Build history of the part. All positions in model axes, mm. Round coordinates to 2 decimals unless told otherwise and drop trailing zeros. Write each loop counter-clockwise with the first axis right and the second up, starting at its lowest first coordinate (ties: lowest second). Pieces come first, ordered by that corner, then holes. Notation, with made-up numbers: M -2,33 L 25,33 A22 ccw 25,72 Z; hole C -32,-23.75 d2. An arc over 180 degrees is marked long. Write item = value, one per line.
from build123d import *

# Parameters (mm, degrees)
BOSS_EXTRUDE1_DEPTH = 3
SKETCH2_R           = 1.5
SKETCH2_W           = 6
SKETCH2_H           = 4
CUT_EXTRUDE1_DEPTH  = 3


with BuildPart() as part:
    # Sketch1 → Boss-Extrude1 (new body)
    with BuildSketch(Plane(origin=(0, 0, 0), x_dir=(1, 0, 0), z_dir=(0, 1, 0))):
        Polygon((-41, -41), (-17.5, -41), (-17.5, -38), (17.5, -38), (17.5, -41), (41, -41), (41, -17.5), (38, -17.5), (38, 17.5), (41, 17.5), (41, 41), (17.5, 41), (17.5, 38), (-17.5, 38), (-17.5, 41), (-41, 41), (-41, 17.5), (-38, 17.5), (-38, -17.5), (-41, -17.5), align=None)
    extrude(amount=BOSS_EXTRUDE1_DEPTH)

    # Sketch2 → Cut-Extrude1 (cut)
    with BuildSketch(Plane(origin=(0, 3, 0), x_dir=(1, 0, 0), z_dir=(0, 1, 0))):
        with Locations((0, -5.5)):
            Circle(SKETCH2_R)
        with Locations((0, 12)):
            Rectangle(SKETCH2_W, SKETCH2_H)
    extrude(amount=-CUT_EXTRUDE1_DEPTH, mode=Mode.SUBTRACT)


solid = part.part
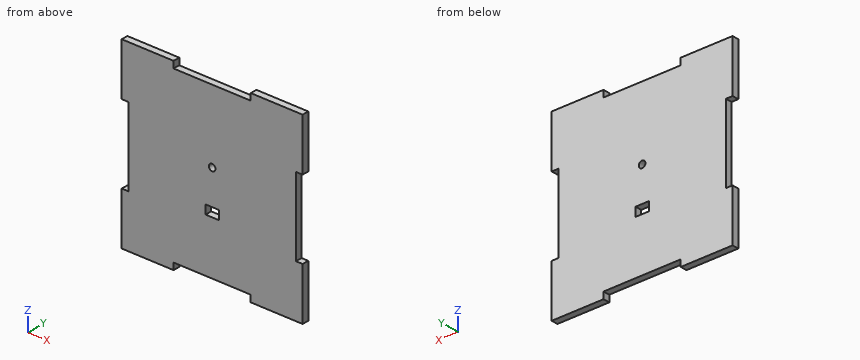
1. Band-saw the part on B-B (x = 0). List the corners of the cut face in (y, z).
Responses:
outline = M 0,-38 L 3,-38 L 3,-14 L 0,-14 Z; M 0,-10 L 3,-10 L 3,4 L 0,4 Z; M 0,7 L 3,7 L 3,38 L 0,38 Z
2. Probe probe 1 along Z at (x, y) = (0, 1.6); probe 2 along X at (y, z) = (2.3, 5.5); probe 3 along Z at (x, y) = (-2.5, 1). List the from-to ranges inside material, lowest first.
Responses:
probe_1 = -38 to -14, -10 to 4, 7 to 38
probe_2 = -38 to -1.5, 1.5 to 38
probe_3 = -38 to -14, -10 to 38
3. Flat gauge pins, fed straight in: pin 1 (1.5 mm diameter, centred on x = -1, y = 1, fed in from +Z); pin 2 (1.5 mm diameter, centred on y = 2, z = -8.5, fed in from +X); pin 3 (0.9 mm diameter, centred on x = 1, y = 2, fed in from -Z). Where does each tip first touch, or does it go through?
Responses:
pin_1 = 38
pin_2 = 38
pin_3 = -38
4. Band-saw the part on A-A (y = 0.5). List the corners of the cut face in (x, z).
Responses:
outline = M -41,-41 L -17.5,-41 L -17.5,-38 L 17.5,-38 L 17.5,-41 L 41,-41 L 41,-17.5 L 38,-17.5 L 38,17.5 L 41,17.5 L 41,41 L 17.5,41 L 17.5,38 L -17.5,38 L -17.5,41 L -41,41 L -41,17.5 L -38,17.5 L -38,-17.5 L -41,-17.5 Z; hole M -3,-14 L 3,-14 L 3,-10 L -3,-10 Z; hole C 0,5.5 d3
5. Band-saw the part on C-C (z = 5.5). List the corners of the cut face in (x, y), plus the area to 3 significant figures.
Responses:
outline = M -38,0 L -1.5,0 L -1.5,3 L -38,3 Z; M 1.5,0 L 38,0 L 38,3 L 1.5,3 Z
area = 219 mm²
6. Band-saw the part on D-D (z = 15.5). List the corners of the cut face in (x, y), plus the area to 3 significant figures.
Responses:
outline = M -38,0 L 38,0 L 38,3 L -38,3 Z
area = 228 mm²
